```python
from build123d import *

# Parameters (mm, degrees)
F1_DEPTH = 44.45
F3_DEPTH = 12.7
F4_W     = 31.75
F4_H     = 13.6071431206
F5_DEPTH = 44.45
F7_START = 54.864
F6_R     = 9.3076399549
F7_DEPTH = 60.706


with BuildPart() as f1:
    # F0 (on Front) → F1 (new body)
    with BuildSketch(Plane.XZ):
        Polygon((13.5610163573, 31.75), (-11.8389836427, 31.75), (-30.8889836427, 12.7), (-30.8889836427, 0), (32.6110163573, 0), (32.6110163573, 12.7), align=None)
    extrude(amount=F1_DEPTH)

    # F2 (on Front) → F3 (join)
    with BuildSketch(Plane.XZ):
        Polygon((18.4121006752, 69.85), (-13.3378993248, 69.85), (-60.8358993248, 22.098), (-60.8358993248, 0), (65.9101006752, 0), (65.9101006752, 22.098), align=None)
    extrude(amount=F3_DEPTH)

    # F4 (on Front) → F5 (join)
    with BuildSketch(Plane.XZ):
        with Locations((1.9634375349, 62.6644603908)):
            Rectangle(F4_W, F4_H)
    extrude(amount=F5_DEPTH)

    # F6 (on Top) → F7 (cut)
    with BuildSketch(Plane.XY.offset(F7_START)):
        with Locations((2.6179165579, -29.2897745967)):
            Circle(F6_R)
    extrude(amount=F7_DEPTH, mode=Mode.SUBTRACT)


solid = f1.part
```
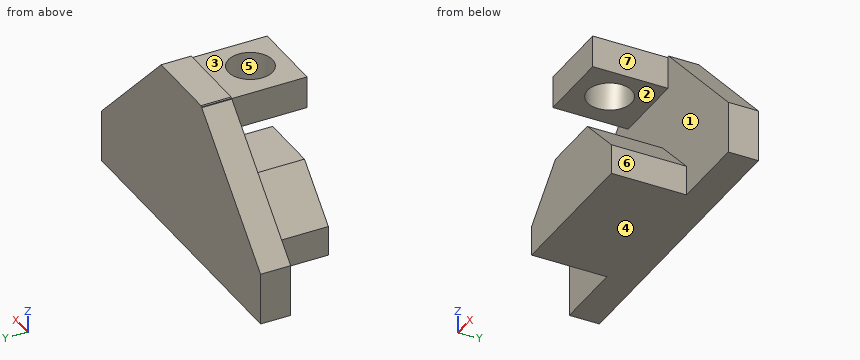
Can you work these out from the model? Positions are in its coordinate system, mm. Face numbers are marked on the shaded views. A direction names the side the tool comes from. Round coordinates to 2 decimals unless told otherwise and drop trailing zeros. Loops run counter-clockwise (first coordinate to the right, second up) from the corner with the lowest first, then second, coordinate; pieces in that order, holes last.
Item 1: Which directions (+Z, -Z, +X, -X, +Y, -Y) give clear straight access to the entire face, cutting with the end or side of a thin tool? Please do the marked faces 5, 6 and 7.
Item 2: Please list where these lines run through material, in increasing order: L1, parallel to Z at x = 10.5, y = -32; L2, parallel to X at y = -28.5, z = 3; L3, parallel to Y at x = -2, z = 57.5.
Item 3: Suppose I cut it at C-C, the plane y = -34.5. Write out the boundary of the cut face in (x, z), then the cut area to 3 significant figures.
Item 4: Will these pins go through, and if not, where does the flat tip stop? pin 1 Ø11 at (x, y) = (2.62, -29.29) entering from +Z; pin 2 Ø8 at (x, y) = (-8.5, -30.5) entering from -Z; pin 3 Ø15 at (y, z) = (-30.5, 64.5) entering from +X; pin 4 Ø10 at (y, z) = (-6.5, 62) entering from +X.
Item 5: If we mould it in two halves opening along Z, with no side actions, what happens to the marked faces 1, 2, 3 and 4? For each: +Z half, -Z half, draft (parallel to the pull), parting line (faces both ways), or undercut.
Item 6: Suppose I cut it at A-A, the plane y = -40.5. Write out the boundary of the cut face in (x, z).
Item 7: Suppose I cut it at B-B, the plane x = 6. Write out the boundary of the cut face in (y, z).
Item 8: Suppose I cut it at D-D, the plane z = 60. Write out the boundary of the cut face in (x, y).
Reported:
1. face 5: +Z
1. face 6: +Z, -Z, +X, -Y
1. face 7: +Z, +X, -Y
2. L1: z = 0 to 31.75
2. L2: x = -30.89 to 32.61
2. L3: y = -44.45 to -37.37, -21.21 to 0
3. outline: (-30.89, 0) - (32.61, 0) - (32.61, 12.7) - (13.56, 31.75) - (-11.84, 31.75) - (-30.89, 12.7) - close; (-13.91, 55.86) - (-5.09, 55.86) - (-5.09, 69.47) - (-13.91, 69.47) - close; (10.33, 55.86) - (17.84, 55.86) - (17.84, 69.47) - (10.33, 69.47) - close
3. area: 1,880 mm2
4. pin 1: stops at z = 31.75
4. pin 2: stops at z = 0
4. pin 3: stops at x = 17.84
4. pin 4: stops at x = 31.19
5. face 1: undercut
5. face 2: undercut
5. face 3: +Z half
5. face 4: -Z half
6. outline: (-30.89, 0) - (32.61, 0) - (32.61, 12.7) - (13.56, 31.75) - (-11.84, 31.75) - (-30.89, 12.7) - close; (-13.91, 55.86) - (17.84, 55.86) - (17.84, 69.47) - (-13.91, 69.47) - close
7. outline: (-44.45, 0) - (0, 0) - (0, 69.85) - (-12.7, 69.85) - (-12.7, 69.47) - (-20.62, 69.47) - (-20.62, 55.86) - (-12.7, 55.86) - (-12.7, 31.75) - (-44.45, 31.75) - close; (-44.45, 55.86) - (-37.96, 55.86) - (-37.96, 69.47) - (-44.45, 69.47) - close
8. outline: (-23.14, -12.7) - (-13.91, -12.7) - (-13.91, -44.45) - (17.84, -44.45) - (17.84, -12.7) - (28.21, -12.7) - (28.21, 0) - (-23.14, 0) - close; hole circle Ø18.62 at (2.62, -29.29)
